CAD build for the part. Positions are in the model's coordinates, mm. A direction names the side the tool comes from. Coordinates: 2 decimals unless noted, no trailing zeros. Write each loop counter-clockwise with the first axis right and the second up, starting at its lowest first coordinate (ties: lowest second). Pieces come first, ordered by that corner, then holes. Notation, with made-up numbers: (16.25, 85) - (74.25, 85) arc R22 cw to (74.25, 96) - close; hole circle Ø7 at (4, 36.25). An arc over 180 degrees is marked (long way). One line per question, with ' | ' between items. Start each with the question number.
1. Band-saw the part on C-C, the plane z = 1.3. Give the number of separate pieces and of enclosed holes in the cut face, then the cut area to 3 significant figures.
2. Band-saw the part on A-A, the plane x = 227. Write the cut outline in (y, z).
3. Probe line 1 (X direction, y = -25, z = 3.75); line 2 (Y direction, x = 190, z = 2.05); line 3 (Y direction, x = 172.5, z = 0.35). List the from-to ranges inside material, lowest first.
4. Two-plate mould, pull along Y, no slides. Class faces 1 (the flat face through (299, 33, 2)), 2 (the flat face through (293, 79.5, 2)): +Y half, -Y half, draft (parallel to the pull), parting line (faces both ways), or undercut.
5. Which spindle directions (+Z, -Z, +X, -X, +Y, -Y) get a long thin tool onto all of the face, cutting with end or side? Do faces 3 (the flat face through (145, 120, 2)), 4 (the flat face through (295, 72, 2)), 5 (the flat face through (205, -24.935, 2)). Say none if no direction does.
6. Band-saw the part on B-B, the plane y = 71.5. Write the cut outline in (x, z), then the cut area to 3 significant figures.
7. Flat gauge pins, fed straight in: P1, Ø2, axis at y = -26.5, z = 3, coming from the -X side; P2, Ø2, axis at x = 297, z = 2, coming from the +Y side; P3, Ø1.5, axis at y = -10, z = 1.5, coming from the +X side. Where does each tip first touch, or does it go through?
from build123d import *

# Parameters (mm, degrees)
SKETCH_1_R      = 2
SKETCH_1_R_2    = 11
SKETCH_1_R_3    = 1.5
SKETCH_1_W      = 8.12
SKETCH_1_H      = 4.129008776
EXTRUDE_1_DEPTH = 4


with BuildPart() as part:
    # 草图1 → 凸台-拉伸1 (new body)
    with BuildSketch(Plane.XY):
        Polygon((145, 46.5), (149, 46.5), (149, 45.15), (151.6, 45.15), (151.6, 46.5), (153.6, 46.5), (153.6, 49.5), (151.6, 49.5), (151.6, 50.85), (149, 50.85), (149, 49.5), (145, 49.5), (145, 59), (141, 59), (141, 67), (145, 67), (145, 76.5), (149, 76.5), (149, 75.15), (151.6, 75.15), (151.6, 76.5), (153.6, 76.5), (153.6, 79.5), (151.6, 79.5), (151.6, 80.85), (149, 80.85), (149, 79.5), (145, 79.5), (145, 89), (141, 89), (141, 97), (145, 97), (145, 106.5), (149, 106.5), (149, 105.15), (151.6, 105.15), (151.6, 106.5), (153.6, 106.5), (153.6, 109.5), (151.6, 109.5), (151.6, 110.85), (149, 110.85), (149, 109.5), (145, 109.5), (145, 123), (145, 130), (295, 130), (295, 123), (295, 109.5), (291, 109.5), (291, 110.85), (288.4, 110.85), (288.4, 109.5), (286.4, 109.5), (286.4, 106.5), (288.4, 106.5), (288.4, 105.15), (291, 105.15), (291, 106.5), (295, 106.5), (295, 97), (299, 97), (299, 89), (295, 89), (295, 79.5), (291, 79.5), (291, 80.85), (288.4, 80.85), (288.4, 79.5), (286.4, 79.5), (286.4, 76.5), (288.4, 76.5), (288.4, 75.15), (291, 75.15), (291, 76.5), (295, 76.5), (295, 67), (299, 67), (299, 59), (295, 59), (295, 49.5), (291, 49.5), (291, 50.85), (288.4, 50.85), (288.4, 49.5), (286.4, 49.5), (286.4, 46.5), (288.4, 46.5), (288.4, 45.15), (291, 45.15), (291, 46.5), (295, 46.5), (295, 37), (299, 37), (299, 29), (295, 29), (295, 19.5), (291, 19.5), (291, 20.85), (288.4, 20.85), (288.4, 19.5), (286.4, 19.5), (286.4, 16.5), (288.4, 16.5), (288.4, 15.15), (291, 15.15), (291, 16.5), (295, 16.5), (295, 7), (299, 7), (299, -1), (295, -1), (295, -10.5), (291, -10.5), (291, -9.15), (288.4, -9.15), (288.4, -10.5), (286.4, -10.5), (286.4, -13.5), (288.4, -13.5), (288.4, -14.85), (291, -14.85), (291, -13.5), (295, -13.5), (295, -27), (295, -34), (145, -34), (145, -27), (145, -13.5), (149, -13.5), (149, -14.85), (151.6, -14.85), (151.6, -13.5), (153.6, -13.5), (153.6, -10.5), (151.6, -10.5), (151.6, -9.15), (149, -9.15), (149, -10.5), (145, -10.5), (145, -1), (141, -1), (141, 7), (145, 7), (145, 16.5), (149, 16.5), (149, 15.15), (151.6, 15.15), (151.6, 16.5), (153.6, 16.5), (153.6, 19.5), (151.6, 19.5), (151.6, 20.85), (149, 20.85), (149, 19.5), (145, 19.5), (145, 29), (141, 29), (141, 37), (145, 37), align=None)
        with Locations((220, 29)):
            Circle(SKETCH_1_R, mode=Mode.SUBTRACT)
        with Locations((220, 48)):
            Circle(SKETCH_1_R_2, mode=Mode.SUBTRACT)
        with Locations((206.564971157, 34.564971157)):
            Circle(SKETCH_1_R, mode=Mode.SUBTRACT)
        with Locations((201, 48)):
            Circle(SKETCH_1_R, mode=Mode.SUBTRACT)
        with Locations((206.564971157, 61.435028843)):
            Circle(SKETCH_1_R, mode=Mode.SUBTRACT)
        with Locations((220, 67)):
            Circle(SKETCH_1_R, mode=Mode.SUBTRACT)
        with Locations((233.435028843, 61.435028843)):
            Circle(SKETCH_1_R, mode=Mode.SUBTRACT)
        with Locations((239, 48)):
            Circle(SKETCH_1_R, mode=Mode.SUBTRACT)
        with Locations((233.435028843, 34.564971157)):
            Circle(SKETCH_1_R, mode=Mode.SUBTRACT)
        with Locations((220, 123)):
            Circle(SKETCH_1_R_3, mode=Mode.SUBTRACT)
        with Locations((250, 123)):
            Circle(SKETCH_1_R_3, mode=Mode.SUBTRACT)
        with Locations((280, 123)):
            Circle(SKETCH_1_R_3, mode=Mode.SUBTRACT)
        with Locations((160, 123)):
            Circle(SKETCH_1_R_3, mode=Mode.SUBTRACT)
        with Locations((190, 123)):
            Circle(SKETCH_1_R_3, mode=Mode.SUBTRACT)
        with Locations((190, -27)):
            Circle(SKETCH_1_R_3, mode=Mode.SUBTRACT)
        with Locations((160, -27)):
            Circle(SKETCH_1_R_3, mode=Mode.SUBTRACT)
        with Locations((280, -27)):
            Circle(SKETCH_1_R_3, mode=Mode.SUBTRACT)
        with Locations((250, -27)):
            Circle(SKETCH_1_R_3, mode=Mode.SUBTRACT)
        with Locations((220, -27)):
            Circle(SKETCH_1_R_3, mode=Mode.SUBTRACT)
        with Locations((200, 8)):
            Circle(SKETCH_1_R, mode=Mode.SUBTRACT)
        with Locations((240, 8)):
            Circle(SKETCH_1_R, mode=Mode.SUBTRACT)
        with Locations((240, 88)):
            Circle(SKETCH_1_R, mode=Mode.SUBTRACT)
        with Locations((200, 88)):
            Circle(SKETCH_1_R, mode=Mode.SUBTRACT)
        with Locations((220, 8)):
            Circle(SKETCH_1_R, mode=Mode.SUBTRACT)
        with Locations((205, -27)):
            Rectangle(SKETCH_1_W, SKETCH_1_H, mode=Mode.SUBTRACT)
        with Locations((175, -27)):
            Rectangle(SKETCH_1_W, SKETCH_1_H, mode=Mode.SUBTRACT)
        with Locations((265, -27)):
            Rectangle(SKETCH_1_W, SKETCH_1_H, mode=Mode.SUBTRACT)
        with Locations((235, -27)):
            Rectangle(SKETCH_1_W, SKETCH_1_H, mode=Mode.SUBTRACT)
        with Locations((235, 123)):
            Rectangle(SKETCH_1_W, SKETCH_1_H, mode=Mode.SUBTRACT)
        with Locations((265, 123)):
            Rectangle(SKETCH_1_W, SKETCH_1_H, mode=Mode.SUBTRACT)
        with Locations((175, 123)):
            Rectangle(SKETCH_1_W, SKETCH_1_H, mode=Mode.SUBTRACT)
        with Locations((205, 123)):
            Rectangle(SKETCH_1_W, SKETCH_1_H, mode=Mode.SUBTRACT)
    extrude(amount=EXTRUDE_1_DEPTH)


solid = part.part
Filled in:
1) separate pieces: 1 | enclosed holes: 32 | area: 23,600 mm²
2) outline: (-34, 0) - (39.51, 0) - (39.51, 4) - (-34, 4) - close; (56.49, 0) - (130, 0) - (130, 4) - (56.49, 4) - close
3) line 1: x = 145 to 170.94, 179.06 to 200.94, 209.06 to 230.94, 239.06 to 260.94, 269.06 to 295 | line 2: y = -34 to -28.5, -25.5 to 121.5, 124.5 to 130 | line 3: y = -34 to -29.06, -24.94 to 120.94, 125.06 to 130
4) face 1: draft | face 2: undercut
5) face 3: +Z, -Z, -X, +Y | face 4: +Z, -Z, +X | face 5: +Z, -Z
6) outline: (145, 0) - (295, 0) - (295, 4) - (145, 4) - close | area: 600 mm²
7) P1: stops at x = 145 | P2: stops at y = 97 | P3: stops at x = 295
